```python
from build123d import *

# Parameters (mm, degrees)
ESTRUSIONE_ESTRUSIONE1_DEPTH = 18
RACCORDO1_R                  = 200


with BuildPart() as part:
    # Schizzo1 → Estrusione-Estrusione1 (new body)
    with BuildSketch(Plane.XY):
        with BuildLine():
            ThreePointArc((-66.988913829, 53.65), (-70.163913829, 56.825), (-66.988913829, 60))
            Line((-66.988913829, 60), (-48.988913829, 60))
            ThreePointArc((-48.988913829, 60), (-45.813913829, 56.825), (-48.988913829, 53.65))
            Line((-48.988913829, 53.65), (-48.988913829, 0.90918463))
            ThreePointArc((-48.988913829, 0.90918463), (-23.132063713, 16.539501058), (-12.988913829, 45))
            ThreePointArc((-12.988913829, 45), (-21.036068748, 70.680483648), (-42.299457846, 87.176308171))
            ThreePointArc((-42.299457846, 87.176308171), (-50.148301569, 88.565285591), (-57.988913829, 90))
            ThreePointArc((-57.988913829, 90), (-102.761040714, 49.52290329), (-66.988913829, 0.90918463))
            Line((-66.988913829, 0.90918463), (-66.988913829, 53.65))
        make_face()
        with BuildLine():
            ThreePointArc((-12.988913829, 45), (-23.132063713, 16.539501058), (-48.988913829, 0.90918463))
            Line((-48.988913829, 0.90918463), (-48.988913829, -1.642858287))
            ThreePointArc((-48.988913829, -1.642858287), (192.011086171, -23.052237245), (433.011086171, -1.642858287))
            Line((433.011086171, -1.642858287), (433.011086171, 0.90918463))
            ThreePointArc((433.011086171, 0.90918463), (397.145771503, 41.520985802), (426.321630188, 87.176308171))
            ThreePointArc((426.321630188, 87.176308171), (192.011086171, 66.947762755), (-42.299457846, 87.176308171))
            ThreePointArc((-42.299457846, 87.176308171), (-21.036068748, 70.680483648), (-12.988913829, 45))
        make_face()
        with BuildLine():
            ThreePointArc((442.011086171, 90), (434.17047391, 88.565285591), (426.321630188, 87.176308171))
            ThreePointArc((426.321630188, 87.176308171), (397.145771503, 41.520985802), (433.011086171, 0.90918463))
            Line((433.011086171, 0.90918463), (433.011086171, 53.65))
            ThreePointArc((433.011086171, 53.65), (429.836086171, 56.825), (433.011086171, 60))
            Line((433.011086171, 60), (451.011086171, 60))
            ThreePointArc((451.011086171, 60), (454.186086171, 56.825), (451.011086171, 53.65))
            Line((451.011086171, 53.65), (451.011086171, 0.90918463))
            ThreePointArc((451.011086171, 0.90918463), (476.867936287, 16.539501058), (487.011086171, 45))
            ThreePointArc((487.011086171, 45), (478.963931252, 70.680483648), (457.700542154, 87.176308171))
            ThreePointArc((457.700542154, 87.176308171), (449.851698431, 88.565285591), (442.011086171, 90))
        make_face()
        with BuildLine():
            ThreePointArc((487.011086171, 45), (476.867936287, 16.539501058), (451.011086171, 0.90918463))
            Line((451.011086171, 0.90918463), (451.011086171, -1.642858287))
            ThreePointArc((451.011086171, -1.642858287), (692.011086171, -23.052237245), (933.011086171, -1.642858287))
            Line((933.011086171, -1.642858287), (933.011086171, 0.90918463))
            ThreePointArc((933.011086171, 0.90918463), (897.145771503, 41.520985802), (926.321630188, 87.176308171))
            ThreePointArc((926.321630188, 87.176308171), (692.011086171, 66.947762755), (457.700542154, 87.176308171))
            ThreePointArc((457.700542154, 87.176308171), (478.963931252, 70.680483648), (487.011086171, 45))
        make_face()
        with BuildLine():
            ThreePointArc((942.011086171, 90), (934.17047391, 88.565285591), (926.321630188, 87.176308171))
            ThreePointArc((926.321630188, 87.176308171), (897.145771503, 41.520985802), (933.011086171, 0.90918463))
            Line((933.011086171, 0.90918463), (933.011086171, 53.65))
            ThreePointArc((933.011086171, 53.65), (929.836086171, 56.825), (933.011086171, 60))
            Line((933.011086171, 60), (951.011086171, 60))
            ThreePointArc((951.011086171, 60), (954.186086171, 56.825), (951.011086171, 53.65))
            Line((951.011086171, 53.65), (951.011086171, 0.90918463))
            ThreePointArc((951.011086171, 0.90918463), (976.867936287, 16.539501058), (987.011086171, 45))
            ThreePointArc((987.011086171, 45), (973.830891324, 76.819805153), (942.011086171, 90))
        make_face()
    extrude(amount=ESTRUSIONE_ESTRUSIONE1_DEPTH)

    # Raccordo1
    raccordo1_edges = [part.edges().sort_by_distance(p)[0] for p in [
        (442.011086171, 90, 9),
    ]]
    fillet(raccordo1_edges, radius=RACCORDO1_R)


solid = part.part
```
Design review of the part built by this model. Coordinates are the model's own, in mm. A direction names the side the tool comes from. Give positions to 0.01 mm unless a question says otherwise; leave off trailing zeros. Write each loop counter-clockwise with the first axis right and the second up, starting at its lowest first coordinate (ties: lowest second). Pieces come first, ordered by that corner, then holes.
(1) Wall thickness on line 1 along X through (y, z) = (29, 14.25); line 2 along X through (y, z) = (24, 2.25); line 3 along Y through (x, z) = (377, 13.5): over which ranges is each line inside the solid? List them lowest first.
Checked values:
line 1: x = -100.05 to -66.99, -48.99 to 433.01, 451.01 to 933.01, 951.01 to 984.07
line 2: x = -97.79 to -66.99, -48.99 to 433.01, 451.01 to 933.01, 951.01 to 981.81
line 3: y = -10.48 to 79.52
(2) Clearance check with flat-ended pins moving along their axes: pin 1 Ø1 at (y, z) = (75, 14.5) entering from +X; pin 2 Ø9 at (y, z) = (34, 9) entering from +X; pin 3 Ø5.5 at (y, z) = (17, 5) entering from -X; pin 4 Ø2 at (x, y) = (528, 69) entering from -Z. State where each tip first meets the part, or that it passes through.
Checked values:
pin 1: stops at x = 975.99
pin 2: stops at x = 986.54
pin 3: stops at x = -95.24
pin 4: stops at z = 0
(3) Mouldability with a two-part tool opening along X and no side actions: class faces 1 (the face through (-102.66, 50.44, 8.87)), 2 (the face through (434, 72, 0)), 3 (the face through (951.011, 28, 9)) as +X half, -X half, draft (parallel to the pull), parting line (faces both ways), or undercut.
Checked values:
face 1: -X half
face 2: draft
face 3: undercut
(4) Add section A-A (y = 29.5). Give the boundary of the cut face in (x, z), and give its area (3 significant figures).
Checked values:
outline: (-100.24, 0) - (-66.99, 0) - (-66.99, 18) - (-100.24, 18) - close; (-48.99, 0) - (433.01, 0) - (433.01, 18) - (-48.99, 18) - close; (451.01, 0) - (933.01, 0) - (933.01, 18) - (451.01, 18) - close; (951.01, 0) - (984.26, 0) - (984.26, 18) - (951.01, 18) - close
area: 18,500 mm2
(5) Tool access review of faces 4 (the face through (434, 72, 18)), 5 (the face through (942, 60, 9)): name each direction out of +Z, -Z, +X, -X, +Y, -Y from which nothing blocks a thin tool from reaching the whole face with its end or side.
Checked values:
face 4: +Z, +X, -X, +Y, -Y
face 5: +Z, -Z, -Y
(6) Add section B-B (x = 571.5). Give the boundary of the cut face in (y, z).
Checked values:
outline: (-17.73, 0) - (72.27, 0) - (72.27, 18) - (-17.73, 18) - close
